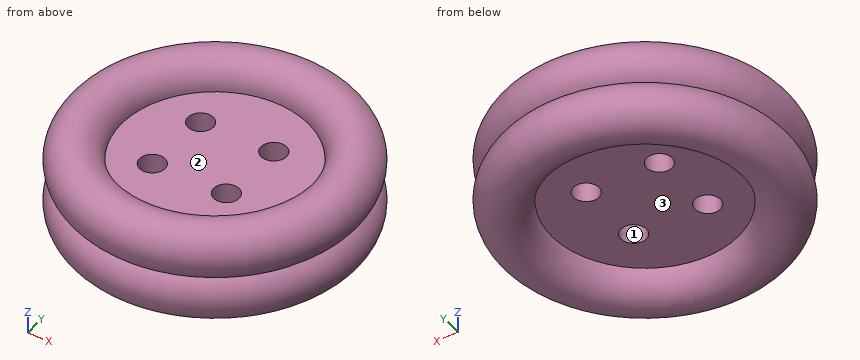
from build123d import *

# Parameters (mm, degrees)
F2_R     = 1.905
F3_DEPTH = 25.4


with BuildPart() as f1:
    # F0 (on Front) → F1 (revolve)
    with BuildSketch(Plane.XZ):
        Polygon((-13.8811003439, 0), (0, 0), (0, 6.5071131103), (-13.8830111907, 6.5071131103), (-17.7800003439, 6.5071131103), (-17.7800003439, 3.8989), (-17.7800003439, 2.6101239571), (-17.7800003439, 0), align=None)
        with BuildLine():
            ThreePointArc((-19.9267050901, 3.2547012063), (-19.6281932552, -3.4330167743), (-13.8811003439, 0))
            Line((-13.8811003439, 0), (-17.7800003439, 0))
            Line((-17.7800003439, 0), (-17.7800003439, 2.6101239571))
            ThreePointArc((-17.7800003439, 2.6101239571), (-18.9006944478, 2.7747453382), (-19.9267050901, 3.2547012063))
        make_face()
        with BuildLine():
            ThreePointArc((-17.7800003439, 3.8989), (-18.9006400444, 3.7343791816), (-19.9267050901, 3.2547012063))
            ThreePointArc((-19.9267050901, 3.2547012063), (-18.9006944478, 2.7747453382), (-17.7800003439, 2.6101239571))
            Line((-17.7800003439, 2.6101239571), (-17.7800003439, 3.8989))
        make_face()
        with BuildLine():
            ThreePointArc((-13.8830111907, 6.5071131103), (-19.6267325049, 9.9387460723), (-19.9267050901, 3.2547012063))
            ThreePointArc((-19.9267050901, 3.2547012063), (-18.9006400444, 3.7343791816), (-17.7800003439, 3.8989))
            Line((-17.7800003439, 3.8989), (-17.7800003439, 6.5071131103))
            Line((-17.7800003439, 6.5071131103), (-13.8830111907, 6.5071131103))
        make_face()
    revolve(axis=Axis((0, 0, 3.2535565551), (0, 0, 1)))

    # F2 (on Top) → F3 (cut)
    with BuildSketch(Plane.XY):
        with Locations((-5.7498575188, 5.3529855795)):
            Circle(F2_R)
        with Locations((5.2605080418, 5.4753227159)):
            Circle(F2_R)
        with Locations((-6.1168693937, -5.0456924364)):
            Circle(F2_R)
        with Locations((5.0158319063, -4.9233548343)):
            Circle(F2_R)
    extrude(amount=F3_DEPTH, mode=Mode.SUBTRACT)


solid = f1.part
The listing builds one solid part. Answer for the finished solid, in the listing's coordinates (mm). Face numbers are marked on the shaded views. A direction names the side the tool comes from. Round coordinates to 2 decimals unless told otherwise and drop trailing zeros. Write each loop counter-clockwise with the first axis right and the second up, starting at its lowest first coordinate (ties: lowest second). Pieces come first, ordered by that corner, then holes. Notation, with made-up numbers: M -39.5,77 L -34.5,77 A28 cw -34.5,106 Z; hole C 50,-8.75 d11. An arc over 180 degrees is marked long. Write each question's results on one line, items separated by ' | '. Start each with the question number.
Item 1: A cutting plane is placed at B-B on z = -2.5. Write down the section's boundary in (x, y).
Item 2: For the marked faces 1, 2 and 3, determine the directions among +Z, -Z, +X, -X, +Y, -Y from which every point of the face is accessible in a straight line to the end or side of a thin tool.
Item 3: A cutting plane is placed at A-A on z = 1.25. Write down the section's boundary in (x, y) (1 decimal), and give its area (3 significant figures).
Item 4: A cutting plane is placed at D-D on z = 4.5. Write down the section's boundary in (x, y) (1 decimal), and give its area (3 significant figures).
Item 5: Straight lines are drawn through the part: L1, parallel to Z at x = -1, y = 17.5; L2, parallel to Y at x = 3, z = 7; L3, parallel to Z at x = -4, y = 12.5. For each, find the intervals that lie inside material, in ascending order. Write a range as [from, to].
Item 6: Flat-ended cylindrical pins translate along their axes: pin 1 Ø3 at (x, z) = (-8, 6) entering from +Y; pin 2 Ø2.5 at (x, y) = (-6.12, -5.05) entering from +Z; pin 3 Ø4.5 at (x, y) = (5.26, 5.48) entering from +Z; pin 4 Ø1.5 at (x, z) = (11, -0.5) entering from +Y. Find the tip coordinate at first contact, or state that the pin passes through.
Item 7: A cutting plane is placed at C-C on x = -7. State how many separate pieces and enclosed holes the cut face has, and give its area (3 significant figures).
Check sheet entries:
1) outline: C 0,0 d41.54; hole C 0,0 d29.58
2) face 1: +Z, -Z | face 2: +Z | face 3: -Z
3) outline: C 0,0 d42.9; hole C -6.1,-5 d3.8; hole C -5.7,5.4 d3.8; hole C 5,-4.9 d3.8; hole C 5.3,5.5 d3.8 | area: 1,400 mm²
4) outline: C 0,0 d42.2; hole C -6.1,-5 d3.8; hole C -5.7,5.4 d3.8; hole C 5,-4.9 d3.8; hole C 5.3,5.5 d3.8 | area: 1,360 mm²
5) L1: [-3.89, 10.4] | L2: [-21.44, -13.59], [13.59, 21.44] | L3: [0, 6.51]
6) pin 1: y = 20.66 | pin 2: through | pin 3: z = 6.51 | pin 4: y = 19.08
7) separate pieces: 3 | enclosed holes: 0 | area: 323 mm²
